Geometry: final body of the model. Coordinates: model frame, mm. Round coordinates to 2 decimals unless told otherwise and drop trailing zeros. Loops run counter-clockwise (first coordinate to the right, second up) from the corner with the lowest first, then second, coordinate; pieces in that order, holes last. Notation, with made-up numbers: (51, -33) - (105, -33) arc R22 ccw to (105, -8) - close; hole circle Ø3 at (-0.75, -7). An arc over 180 degrees is marked (long way). Answer as a JSON object with one key per item and string values. Group by question number.
Item 1: First-contact query: pin 1 (6 mm diameter, centred on x = 2.5, z = -10, fed in from -Y); pin 2 (5 mm diameter, centred on x = -1.5, z = -10, fed in from +Y); pin 3 (1.5 mm diameter, centred on x = -2, z = 12, fed in from -Y). Flat tips, straight axial feed; report the tip coordinate or a pass-through.
Item 2: Line query: line 1 (Z direction, x = -1.5, y = 5.75); line 2 (Z direction, x = -3.75, y = 2.5); line 3 (Y direction, x = -7.25, z = 38). Output: solid intervals per line, ascending.
Item 3: Section C-C (z = -53). Return the cut outline in (x, y).
Item 4: Section D-D (y = 4.5). Return the cut outline in (x, z), plus the area to 3 significant figures.
Item 5: Section A-A (x = 0). Return the cut outline in (y, z).
```python
from build123d import *

# Parameters (mm, degrees)
SKETCH1_R               = 2
BOSS_EXTRUDE1_DEPTH     = 40
BOSS_EXTRUDE2_START     = 60
SKETCH5_R               = 2
BOSS_EXTRUDE2_DEPTH     = 60
CUT_EXTRUDE1_DEPTH      = 62.485770712
CUT_EXTRUDE1_DEPTH_BACK = 62.485770712


with BuildPart() as part:
    # Sketch1 → Boss-Extrude1 (new body)
    with BuildSketch(Plane.XY):
        Circle(SKETCH1_R)
    extrude(amount=BOSS_EXTRUDE1_DEPTH)

    # Sketch2 → Revolve1 (revolve)
    with BuildSketch(Plane(origin=(0, 0, 0), x_dir=(1, 0, 0), z_dir=(0, 1, 0))):
        with BuildLine():
            Line((-9.5, -40), (9.5, -40))
            ThreePointArc((9.5, -40), (0, -30.5), (-9.5, -40))
        make_face()
    revolve(axis=Axis((-9.5, 0, 40), (1, 0, 0)))

    # Sketch5 → Boss-Extrude2 (add)
    with BuildSketch(Plane(origin=(0, 0, 0), x_dir=(-1, 0, 0), z_dir=(0, 0, -1)).offset(BOSS_EXTRUDE2_START)):
        Circle(SKETCH5_R)
    extrude(amount=-BOSS_EXTRUDE2_DEPTH)

    # Sketch6 → Cut-Extrude1 (cut, two sides: drawn at the far end of the back side and taken through both)
    with BuildSketch(Plane(origin=(0, 0, 0), x_dir=(0, 0, -1), z_dir=(1, 0, 0)).offset(-CUT_EXTRUDE1_DEPTH_BACK)):
        Polygon((-46.5, 0), (-46.5, 12.012765668), (-54.329815316, 12.012765668), (-54.329815316, -12.092015027), (-46.5, -12.092015027), align=None)
    extrude(amount=CUT_EXTRUDE1_DEPTH + CUT_EXTRUDE1_DEPTH_BACK, mode=Mode.SUBTRACT)


solid = part.part
```
Values:
{
 "1": {"pin 1": "stops at y = -2", "pin 2": "stops at y = 2", "pin 3": "stops at y = -1.56"},
 "2": {"line 1": "z = 32.59 to 46.5", "line 2": "z = 31.64 to 46.5", "line 3": "y = -5.8 to 5.8"},
 "3": {"outline": "circle Ø4 at (0, 0)"},
 "4": {"outline": "(-5.27, 46.5) arc R8.37 ccw (long way) to (5.27, 46.5) - close", "area": "206 mm^2"},
 "5": {"outline": "(-6.93, 46.5) arc R9.5 ccw to (-2, 30.71) - (-2, -60) - (2, -60) - (2, 30.71) arc R9.5 ccw to (6.93, 46.5) - close"}
}
